```python
from build123d import *

# Parameters (mm, degrees)
SKETCH158_W   = 114
SKETCH158_H   = 89
SKETCH158_W_2 = 10.8
SKETCH158_H_2 = 5.6
SKETCH158_W_3 = 10.7
SKETCH158_H_3 = 6.75
PAD_DEPTH     = 4
PAD001_DEPTH  = 2
FILLET_R      = 0.5
SKETCH160_W   = 1.5
SKETCH160_H   = 3
SKETCH160_W_2 = 2.5
SKETCH160_H_2 = 0.9
PAD003_DEPTH  = 104
SKETCH161_R   = 1.4
POCKET_DEPTH  = 5


with BuildPart() as part:
    # Sketch158 → Pad (new body)
    with BuildSketch(Plane.XY):
        with Locations((57, 44.5)):
            Rectangle(SKETCH158_W, SKETCH158_H)
        with Locations((31.2, 52.8)):
            Rectangle(SKETCH158_W_2, SKETCH158_H_2, mode=Mode.SUBTRACT)
        with Locations((47, 52.8)):
            Rectangle(SKETCH158_W_2, SKETCH158_H_2, mode=Mode.SUBTRACT)
        with Locations((15.4, 52.8)):
            Rectangle(SKETCH158_W_2, SKETCH158_H_2, mode=Mode.SUBTRACT)
        with Locations((15.35, 73.375)):
            Rectangle(SKETCH158_W_3, SKETCH158_H_3, mode=Mode.SUBTRACT)
    extrude(amount=PAD_DEPTH)

    # Sketch159 → Pad001 (join)
    with BuildSketch(Plane(origin=(0, 0, 0), x_dir=(1, 0, 0), z_dir=(0, 0, -1))):
        Polygon((70.999116, -84.5074), (85.999116, -84.5074), (102.903847, -48.255089), (76.823852, -55.24321), (91.244924, -31.24253), (92.473681, -36.280333), (98.788067, -17.050922), (82.960377, -29.532091), (88.686929, -29.085032), (65.175526, -61.445717), (92.221447, -54.198777), align=None)
    extrude(amount=PAD001_DEPTH)

    # Fillet
    fillet_edges = [part.edges().sort_by_distance(p)[0] for p in [
        (94.451481, 66.381245, -2),
        (78.499116, 84.5074, -2),
        (81.610281, 69.353088, -2),
        (78.698487, 57.822247, -2),
        (89.86385, 51.74915, -2),
        (84.034388, 43.24287, -2),
        (91.859302, 33.761432, -2),
        (95.630874, 26.665627, -2),
        (90.874222, 23.291507, -2),
        (85.823653, 29.308561, -2),
        (76.931228, 45.265374, -2),
    ]]
    fillet(fillet_edges, radius=FILLET_R)

    # Sketch160 → Pad003 (join)
    with BuildSketch(Plane.YZ):
        with Locations((5.75, 5.5)):
            Rectangle(SKETCH160_W, SKETCH160_H)
        with Locations((5.75, 7.45)):
            Rectangle(SKETCH160_W_2, SKETCH160_H_2)
    extrude(amount=PAD003_DEPTH)

    # Sketch161 → Pocket (cut)
    with BuildSketch(Plane.XY):
        with Locations((107, 7)):
            Circle(SKETCH161_R)
    extrude(amount=POCKET_DEPTH, mode=Mode.SUBTRACT)


solid = part.part
```
Geometry: final body of the model. Coordinates: model frame, mm. A direction names the side the tool comes from. Round coordinates to 2 decimals unless told otherwise and drop trailing zeros. Order: outer loops, then holes, each group sorted by start corner. A loop starts at its lowest first (then second) coordinate and runs counter-clockwise, first axis right, second up. Notation, with made-up numbers: (26, 8) - (31, 8) arc R20 ccw to (31, 44) - close; hole circle Ø7 at (-1.75, 9). An arc over 180 degrees is marked (long way). Use CSV: the item, a comma, the result in double quotes. Start each with the question number.
Q1. Mould query, pull axis X, two halves, no side actions, for faces 6 (the face through (56, 0, 2)), 7 (the face through (95.587, 26.8, -0.74)), 8 (the face through (15, 55.6, 2)). Classes: +X half, -X half, draft (parallel to the pull), parting line (faces both ways), or undercut.
Q2. Section query A-A (z = 1.5). Return loops of the section in (x, y), and give its area (3 significant figures).
Q3. First-contact query: pin 1 (4.5 mm diameter, centred on y = 72.5, z = 2, fed in from -X); pin 2 (1 mm diameter, centred on x = 66, z = 7.5, fed in from +Y); pin 3 (4 mm diameter, centred on x = 70.5, y = 45, fed in from +Z); pin 4 (0.5 mm diameter, centred on x = 75, z = 7.5, fed in from -Y). Flat tips, straight axial feed; report the tip coordinate or a pass-through.
Q4. Section query B-B (x = 107). Return loops of the section in (y, z), and give its area (3 significant figures).
Q5. Access query for faces 1 (the face through (95.54, 26.49, -1.85)), 2 (the face through (51, 6, 7.9)), 3 (the face through (47, 55.6, 2)), 4 (the face through (90.99, 23.2, -0.74)), 5 (the face through (79.524, 57.454, -1.85)). Directions: +Z, -Z, +X, -X, +Y, -Y. A direction counts if a zero-diameter tool reaches every point of the face in a straight line with its end or side. Return the directions, or none.
Q6. Material intervals for line 1 along X through (y, z) = (7, 1.6); line 2 along Y through (x, z) = (107, 1.1); line 3 along Y through (x, z) = (44, 3.75), sorted ascending. Write a range as from..to.
Result set:
1,face 6,"draft"
1,face 7,"+X half"
1,face 8,"undercut"
2,outline,"(0, 0) - (114, 0) - (114, 89) - (0, 89) - close; hole (10, 50) - (20.8, 50) - (20.8, 55.6) - (10, 55.6) - close; hole (10, 70) - (20.7, 70) - (20.7, 76.75) - (10, 76.75) - close; hole (25.8, 50) - (36.6, 50) - (36.6, 55.6) - (25.8, 55.6) - close; hole (41.6, 50) - (52.4, 50) - (52.4, 55.6) - (41.6, 55.6) - close; hole circle Ø2.8 at (107, 7)"
2,area,"9,890 mm2"
3,pin 1,"stops at x = 0"
3,pin 2,"stops at y = 7"
3,pin 3,"stops at z = 4"
3,pin 4,"stops at y = 4.5"
4,outline,"(0, 0) - (5.6, 0) - (5.6, 4) - (0, 4) - close; (8.4, 0) - (89, 0) - (89, 4) - (8.4, 4) - close"
4,area,"345 mm2"
5,face 1,"-Z, +X"
5,face 2,"+Z, +X, -X, +Y, -Y"
5,face 3,"+Z, -Z"
5,face 4,"-Z, -X, -Y"
5,face 5,"-Z"
6,line 1,"x = 0..105.6, 108.4..114"
6,line 2,"y = 0..5.6, 8.4..89"
6,line 3,"y = 0..50, 55.6..89"
